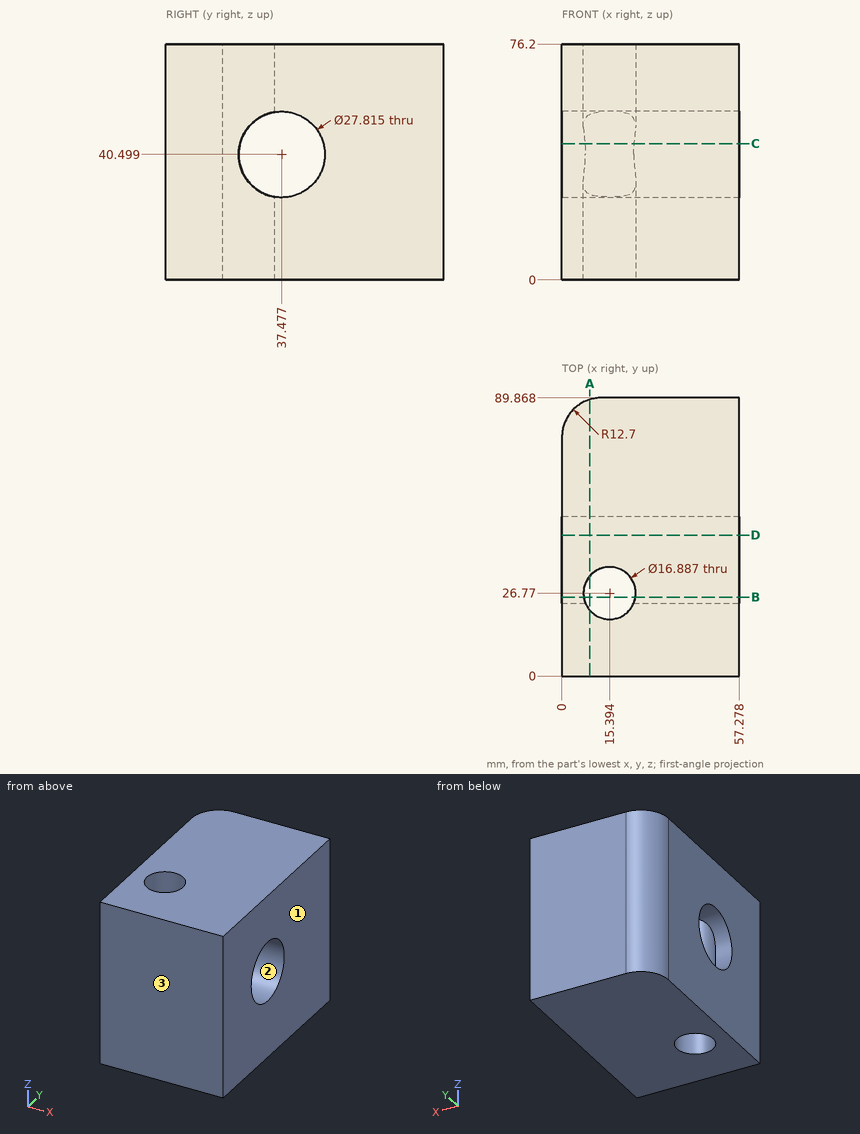
For this review, use the dimensioned drawing (mm, ordinates from the lowest corner) and the shaded views. Round coordinates to 2 decimals unless told otherwise and drop trailing zeros. Write each loop counter-clockwise with the first axis right and the second up, starting at its lowest first coordinate (ties: lowest second). Pieces come first, ordered by that corner, then holes. Notation, with made-up numbers: (3.5, 39.5) - (60.5, 39.5) arc R28 ccw to (60.5, 61.5) - close; hole circle Ø9 at (9.5, -31). An arc over 180 degrees is marked (long way). Use CSV: the item, a comma, the result in double quotes.
1) Add section D-D on y = 45.5. Write out the cut boundary in (x, z), and give its area (3 significant figures).
Conclusion:
outline,"(0, 0) - (57.28, 0) - (57.28, 29.14) - (0, 29.14) - close; (0, 51.86) - (57.28, 51.86) - (57.28, 76.2) - (0, 76.2) - close"
area,"3,060 mm^2"
2) Add section A-A on x = 9. Write out the cut boundary in (y, z) (1 decimal), and give its area (3 significant figures).
Conclusion:
outline,"(0, 0) - (21.3, 0) - (21.3, 76.2) - (0, 76.2) - close; (32.3, 0) - (89.3, 0) - (89.3, 76.2) - (32.3, 76.2) - (32.3, 53.4) arc R13.9 cw (long way) to (32.3, 27.6) - close"
area,"5,520 mm^2"
3) Clearance check with a flat-ended pin moving along its axis: pin 1 Ø10 at (y, z) = (37, 45) entering from +X. State where the tip first meets the part, or that it passes through.
Conclusion:
pin 1,"passes through"
4) Add section B-B on y = 25.5. Write out the cut boundary in (x, z), and give its area (3 significant figures).
Conclusion:
outline,"(0, 0) - (7.05, 0) - (7.05, 33.43) - (0, 33.43) - close; (0, 47.57) - (7.05, 47.57) - (7.05, 76.2) - (0, 76.2) - close; (23.74, 0) - (57.28, 0) - (57.28, 33.43) - (23.74, 33.43) - close; (23.74, 47.57) - (57.28, 47.57) - (57.28, 76.2) - (23.74, 76.2) - close"
area,"2,520 mm^2"
5) Add section C-C on z = 44. Write out the cut boundary in (x, y) (1 decimal), and give its area (3 significant figures).
Conclusion:
outline,"(0, 0) - (57.3, 0) - (57.3, 24) - (23.4, 24) arc R8.4 cw to (7.4, 24) - (0, 24) - close; (0, 50.9) - (57.3, 50.9) - (57.3, 89.9) - (12.7, 89.9) arc R12.7 ccw to (0, 77.2) - close"
area,"3,500 mm^2"
6) The part is to be moulded in two halves that separate along Y. For the marked faces 1, 2 and 3, say which applies: pulls with the +Y half, pulls with the -Y half, needs draft (parallel to the pull), parting line crosses it, or undercut.
Conclusion:
face 1,"needs draft"
face 2,"undercut"
face 3,"pulls with the -Y half"
7) Wall thickness on line 1 along Y through (x, z) = (32.5, 42); line 2 along Z through (x, y) = (16.5, 47.5); line 3 along Y through (x, z) = (13.5, 22): over which ranges is each line inside the solid? List them lowest first. Write a range as from..to.
Conclusion:
line 1,"y = 0..23.65, 51.3..89.87"
line 2,"z = 0..30.86, 50.14..76.2"
line 3,"y = 0..18.54, 35..89.87"
